The model under review builds one solid part; all positions refer to its coordinate system, in mm. A direction names the side the tool comes from. Coordinates: 2 decimals unless noted, no trailing zeros. Write each loop counter-clockwise with the first axis right and the second up, starting at its lowest first coordinate (ties: lowest second). Pieces come first, ordered by that corner, then holes. Notation, with made-up numbers: (-8, 33) - (2, 33) arc R14 cw to (2, 39) - close; hole circle Ø5 at (79.5, 6). An arc over 180 degrees is marked (long way). Put each result on its own line as item: value.
from build123d import *

# Parameters (mm, degrees)
F0_R     = 4.5
F1_DEPTH = 15
F3_DEPTH = 10.5


with BuildPart() as f1:
    # F0 (on Front) → F1 (new body)
    with BuildSketch(Plane.XZ):
        with BuildLine():
            Line((40, 50), (-40, 50))
            ThreePointArc((-40, 50), (-47.071068, 47.071068), (-50, 40))
            Line((-50, 40), (-50, -40))
            ThreePointArc((-50, -40), (-47.071068, -47.071068), (-40, -50))
            Line((-40, -50), (40, -50))
            ThreePointArc((40, -50), (47.071068, -47.071068), (50, -40))
            Line((50, -40), (50, 40))
            ThreePointArc((50, 40), (47.071068, 47.071068), (40, 50))
        make_face()
        with Locations((-39, -38)):
            Circle(F0_R, mode=Mode.SUBTRACT)
        with Locations((39, -38)):
            Circle(F0_R, mode=Mode.SUBTRACT)
        with Locations((-39, 38)):
            Circle(F0_R, mode=Mode.SUBTRACT)
        with Locations((39, 38)):
            Circle(F0_R, mode=Mode.SUBTRACT)
    extrude(amount=F1_DEPTH)

    # F2 (on face) → F3 (cut)
    with BuildSketch(Plane(origin=(0, 0, 0), x_dir=(-1, 0, 0), z_dir=(0, 1, 0))):
        Polygon((-25, 14.751212), (-25, -50), (25, -50), (25, 29.937138), (-25, 30), align=None)
    extrude(amount=-F3_DEPTH, mode=Mode.SUBTRACT)


solid = f1.part
1. Machinability: for faces 1 (the cylindrical face through (-36.92, -7.4, -41.99)), 2 (the flat face through (0, -10.5, -9)), which of the approach directions +Z, -Z, +X, -X, +Y, -Y give a long, thin tool a straight path to every point of the face, cutting with its end or side? Answer none if there is none.
Determined:
face 1: +Y, -Y
face 2: -Z, +Y
2. Consider section D-D on z = -38. State the section outline as (x, y) points, plus the area to 3 significant figures.
Determined:
outline: (-50, -15) - (-43.5, -15) - (-43.5, 0) - (-50, 0) - close; (-34.5, -15) - (34.5, -15) - (34.5, 0) - (25, 0) - (25, -10.5) - (-25, -10.5) - (-25, 0) - (-34.5, 0) - close; (43.5, -15) - (50, -15) - (50, 0) - (43.5, 0) - close
area: 705 mm^2
3. The part is to be moulded in two halves that separate along X. For faces 3 (the flat face through (-25, -5, -11)), 4 (the flat face through (-1, -15, 1)), 5 (the cylindrical face through (-46.99, -7.4, 47.15)), say which applies: +X half, -X half, draft (parallel to the pull), parting line (faces both ways), or undercut.
Determined:
face 3: undercut
face 4: draft
face 5: -X half
4. Consider section A-A on z = 38. State the section outline as (x, y) points, plus the area to 3 significant figures.
Determined:
outline: (-50, -15) - (-43.5, -15) - (-43.5, 0) - (-50, 0) - close; (-34.5, -15) - (34.5, -15) - (34.5, 0) - (-34.5, 0) - close; (43.5, -15) - (50, -15) - (50, 0) - (43.5, 0) - close
area: 1,230 mm^2
5. Consider section C-C on y = -2.5. State the section outline as (x, z) points.
Determined:
outline: (-50, -40) arc R10 ccw to (-40, -50) - (-25, -50) - (-25, 29.94) - (25, 30) - (25, -50) - (40, -50) arc R10 ccw to (50, -40) - (50, 40) arc R10 ccw to (40, 50) - (-40, 50) arc R10 ccw to (-50, 40) - close; hole circle Ø9 at (-39, -38); hole circle Ø9 at (-39, 38); hole circle Ø9 at (39, -38); hole circle Ø9 at (39, 38)
6. For pin 1 Ø2 at (x, y) = (16, -9) entering from -Z; pin 2 Ø15 at (x, z) = (3, -22.5) entering from +Y, all flat-tipped, find the tip position at first contact; note any pin that passes through.
Determined:
pin 1: stops at z = 29.99
pin 2: stops at y = -10.5
7. Consider section B-B on x = 36.5. State the section outline as (y, z) points.
Determined:
outline: (-15, -50) - (0, -50) - (0, -41.74) - (-15, -41.74) - close; (-15, -34.26) - (0, -34.26) - (0, 34.26) - (-15, 34.26) - close; (-15, 41.74) - (0, 41.74) - (0, 50) - (-15, 50) - close
8. To check wall thickness, follow probe 1 along Z at (x, y) = (-39, -10.5); probe 2 along X at (y, z) = (-0.75, -3.5); probe 3 along X at (y, z) = (-2.75, 40.5). State the ranges of each line that lie inside material, in increasing order.
Determined:
probe 1: z = -50 to -42.5, -33.5 to 33.5, 42.5 to 50
probe 2: x = -50 to -25, 25 to 50
probe 3: x = -49.99 to -42.74, -35.26 to 35.26, 42.74 to 49.99
